```python
from build123d import *

# Parameters (mm, degrees)
F0_R     = 13.323828
F1_DEPTH = 25.4
F2_R     = 12.7


with BuildPart() as f1:
    # F0 (on Top) → F1 (new body)
    with BuildSketch(Plane.XY):
        with BuildLine():
            Line((-10.201276, 15.701963), (-49.335584, 15.701963))
            ThreePointArc((-49.335584, 15.701963), (-52.774252, -9.280166), (-49.655831, -34.304287))
            Line((-49.655831, -34.304287), (55.006877, -34.304287))
            Line((55.006877, -34.304287), (55.006877, -5.300662))
            Line((55.006877, -5.300662), (20.602578, 33.70421))
            Line((20.602578, 33.70421), (-10.201276, 33.70421))
            Line((-10.201276, 33.70421), (-10.201276, 15.701963))
        make_face()
        with Locations((37.604701, -15.301912)):
            Circle(F0_R, mode=Mode.SUBTRACT)
    extrude(amount=F1_DEPTH)

    # F2
    f2_edges = [f1.edges().sort_by_distance(p)[0] for p in [
        (-49.655831, -34.304287, 12.7),
    ]]
    fillet(f2_edges, radius=F2_R)


solid = f1.part
```
The model under review builds one solid part; all positions refer to its coordinate system, in mm. A direction names the side the tool comes from. Round coordinates to 2 decimals unless told otherwise and drop trailing zeros. Loops run counter-clockwise (first coordinate to the right, second up) from the corner with the lowest first, then second, coordinate; pieces in that order, holes last. Notation, with made-up numbers: (-5, 75.5) -> (37, 75.5) arc R16 cw to (37, 95.5) -> close; hole circle Ø7 at (16, 45.5). An arc over 180 degrees is marked (long way). Answer as a JSON object with one key per item and string values. Group by question number.
1) We need section C-C on z = 15.5. Write out the cut boundary in (x, y), then the cut area to 3 significant figures.
2) For pin 1 Ø9 at (y, z) = (21.5, 18) entering from -X; pin 2 Ø10 at (y, z) = (-23, 13.5) entering from -X; pin 3 Ø1 at (y, z) = (4.5, 3) entering from +X, all flat-tipped, find the tip position at first contact; note any pin that passes through.
3) We need section B-B on x = 30.5. Write out the cut boundary in (y, z).
4) We need section D-D on x = -16.5. Write out the cut boundary in (y, z), then the cut area to 3 significant figures.
5) We need section A-A on y = -26. Write out the cut boundary in (x, z), then the cut area to 3 significant figures.
6) Mouldability with a two-part tool opening along X and no side actions: class faces 3 (the face through (24.294, -14.716, 12.522)), 4 (the face through (-47.689, -31.104, 12.878)), 5 (the face through (38.046, 13.929, 12.522)), 6 (the face through (7, -34.304, 13)) as released by +X, released by -X, zero draft, split by the parting line, or undercut.
7) For line 1 (Y direction, x = -23, z = 17.5); line 2 (X direction, y = -11.5, z = 13); line 3 (X direction, y = -20, z = 14.75), list the stretches that pass through material, from the lowest coordinate up. Write a range as [from, to].
8) For faces 1 (the face through (-52.56, -3.43, 12.52)), 2 (the face through (-29, 15.702, 13)), list the 3-axis set-ups (+Z, -Z, +X, -X, +Y, -Y) from which the entire face can be reached by the end or side of a thin tool; tool diameter is ignored.
Result set:
{
 "1": {"outline": "(-51.84, -23.37) arc R12.7 ccw to (-39.26, -34.3) -> (55.01, -34.3) -> (55.01, -5.3) -> (20.6, 33.7) -> (-10.2, 33.7) -> (-10.2, 15.7) -> (-49.34, 15.7) arc R96.98 ccw to start; hole circle Ø26.65 at (37.6, -15.3)", "area": "5,260 mm²"},
 "2": {"pin 1": "x = -10.2", "pin 2": "x = -52.44", "pin 3": "x = 46.8"},
 "3": {"outline": "(-34.3, 0) -> (-26.57, 0) -> (-26.57, 25.4) -> (-34.3, 25.4) -> close; (-4.03, 0) -> (22.48, 0) -> (22.48, 25.4) -> (-4.03, 25.4) -> close"},
 "4": {"outline": "(-34.3, 0) -> (15.7, 0) -> (15.7, 25.4) -> (-34.3, 25.4) -> close", "area": "1,270 mm²"},
 "5": {"outline": "(-51.17, 0) -> (29.66, 0) -> (29.66, 25.4) -> (-51.17, 25.4) -> close; (45.55, 0) -> (55.01, 0) -> (55.01, 25.4) -> (45.55, 25.4) -> close", "area": "2,290 mm²"},
 "6": {"face 3": "undercut", "face 4": "released by -X", "face 5": "released by +X", "face 6": "zero draft"},
 "7": {"line 1": "[-34.3, 15.7]", "line 2": "[-52.76, 24.83], [50.37, 55.01]", "line 3": "[-52.25, 25.14], [50.07, 55.01]"},
 "8": {"face 1": "+Z, -Z, -X", "face 2": "+Z, -Z, -X, +Y"}
}
